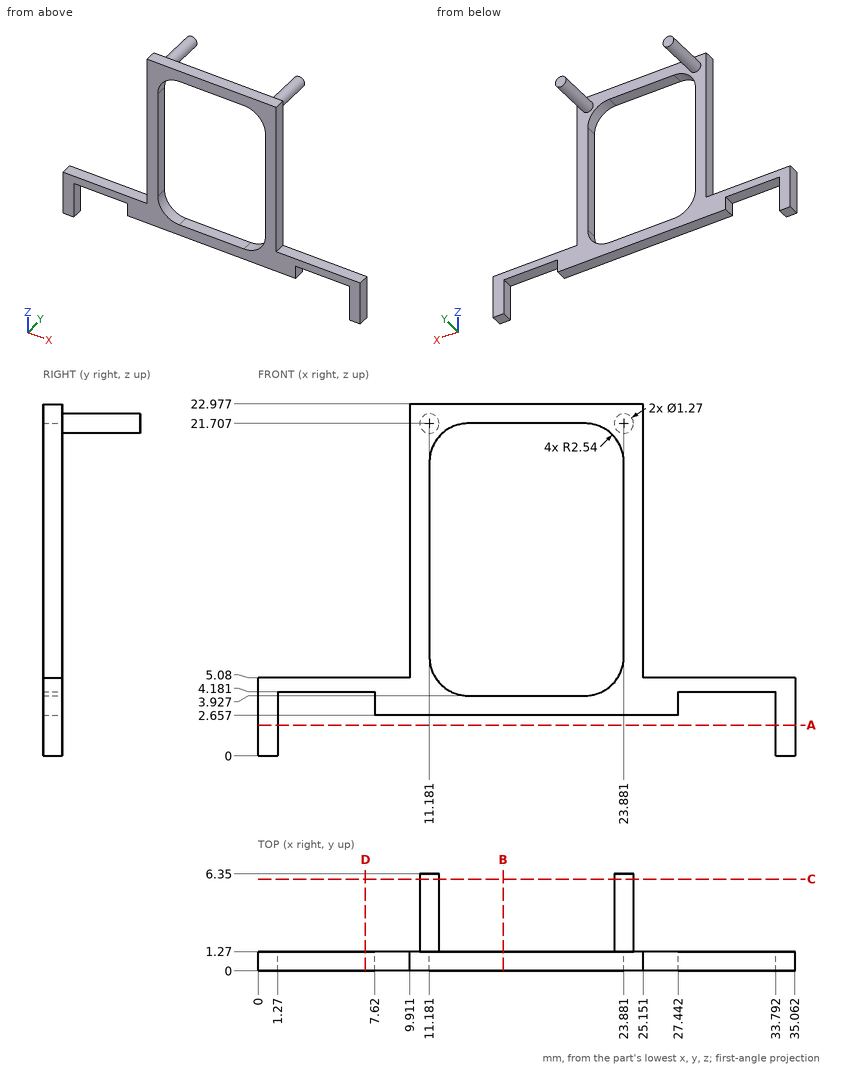
Verification items for this drawing (mm, ordinates from the low corner). Give positions to 0.01 mm unless a question says otherwise; leave off trailing zeros. Write each loop counter-clockwise with the first axis right and the second up, starting at its lowest first coordinate (ties: lowest second). Pieces come first, ordered by that corner, then holes.
1) Section check D-D, the plane x = 7. Record the boundary of the cut face in (y, z).
2) Section check A-A, the plane z = 2. Record the boundary of the cut face in (x, y).
3) Gauge pin test, flat ends, axial feed: pin 1 (1 mm diameter, centred on x = 5, y = 0.5, fed in from -Z); pin 2 (11.5 mm diameter, centred on x = 25, z = 7.5, fed in from +Y); pin 3 (1.4 mm diameter, centred on x = 17.5, y = 0.5, fed in from -Z). Record the tip position at first contact, or that the pin passes through.
4) Section check B-B, the plane x = 16. Record the boundary of the cut face in (y, z).
5) Section check C-C, the plane y = 6. Record the boundary of the cut face in (x, z) (1 decimal).
6) Material ranges on L1, parallel to X at y = 1, z = 16; L2, parallel to Z at x = 19, y = 0.5; L3, parallel to X at y = 4.5, z = 21.25 (1 decimal), recorded low to high.
Computed:
1. outline: (0, 4.18) - (1.27, 4.18) - (1.27, 5.08) - (0, 5.08) - close
2. outline: (0, 0) - (1.27, 0) - (1.27, 1.27) - (0, 1.27) - close; (33.79, 0) - (35.06, 0) - (35.06, 1.27) - (33.79, 1.27) - close
3. pin 1: stops at z = 4.18
3. pin 2: stops at y = 1.27
3. pin 3: stops at z = 2.66
4. outline: (0, 2.66) - (1.27, 2.66) - (1.27, 3.93) - (0, 3.93) - close; (0, 21.71) - (1.27, 21.71) - (1.27, 22.98) - (0, 22.98) - close
5. outline: circle Ø1.3 at (11.2, 21.7); circle Ø1.3 at (23.9, 21.7)
6. L1: x = 9.91 to 11.18, 23.88 to 25.15
6. L2: z = 2.66 to 3.93, 21.71 to 22.98
6. L3: x = 10.7 to 11.6, 23.4 to 24.3
